```python
from build123d import *

# Parameters (mm, degrees)
F1_DEPTH = 520.7
F2_W     = 1016
F2_H     = 53.34
F3_DEPTH = 7.62
F4_R     = 7.62
F5_DEPTH = 10.16
F6_R     = 7.62
F7_DEPTH = 19.05
F8_R     = 7.62
F9_DEPTH = 19.05
F10_SIZE = 5.08


with BuildPart() as f1:
    # F0 (on Right) → F1 (new body, symmetric)
    with BuildSketch(Plane.YZ):
        Polygon((41.91, 39.37), (0, 39.37), (0, 0), (0, -39.37), (41.91, -39.37), (86.868, -26.67), (86.868, 0), (86.868, 26.67), align=None)
    extrude(amount=F1_DEPTH, both=True)

    # F2 (on face) → F3 (cut)
    with BuildSketch(Plane.XZ):
        Rectangle(F2_W, F2_H)
    extrude(amount=-F3_DEPTH, mode=Mode.SUBTRACT)

    # F4 (on face) → F5 (cut)
    with BuildSketch(Plane.XZ.offset(-7.62)):
        with Locations((-488.95, 13.97)):
            Circle(F4_R)
        with Locations((-463.8758824825, 13.97)):
            Circle(F4_R)
        with Locations((-438.8017649651, 13.97)):
            Circle(F4_R)
        with Locations((-413.7276474476, 13.97)):
            Circle(F4_R)
        with Locations((-388.6535299301, 13.97)):
            Circle(F4_R)
        with Locations((-363.5794124126, 13.97)):
            Circle(F4_R)
        with Locations((-338.5052948952, 13.97)):
            Circle(F4_R)
        with Locations((-313.4311773777, 13.97)):
            Circle(F4_R)
        with Locations((-288.3570598602, 13.97)):
            Circle(F4_R)
        with Locations((-263.2829423428, 13.97)):
            Circle(F4_R)
        with Locations((-238.2088248253, 13.97)):
            Circle(F4_R)
        with Locations((-213.1347073078, 13.97)):
            Circle(F4_R)
        with Locations((-188.0605897903, 13.97)):
            Circle(F4_R)
        with Locations((-162.9864722729, 13.97)):
            Circle(F4_R)
        with Locations((-137.9123547554, 13.97)):
            Circle(F4_R)
        with Locations((-112.8382372379, 13.97)):
            Circle(F4_R)
        with Locations((-87.7641197205, 13.97)):
            Circle(F4_R)
        with Locations((-62.690002203, 13.97)):
            Circle(F4_R)
        with Locations((-37.6158846855, 13.97)):
            Circle(F4_R)
        with Locations((-12.541767168, 13.97)):
            Circle(F4_R)
        with Locations((12.5323503494, 13.97)):
            Circle(F4_R)
        with Locations((37.6064678669, 13.97)):
            Circle(F4_R)
        with Locations((62.6805853844, 13.97)):
            Circle(F4_R)
        with Locations((87.7547029018, 13.97)):
            Circle(F4_R)
        with Locations((112.8288204193, 13.97)):
            Circle(F4_R)
        with Locations((137.9029379368, 13.97)):
            Circle(F4_R)
        with Locations((162.9770554543, 13.97)):
            Circle(F4_R)
        with Locations((188.0511729717, 13.97)):
            Circle(F4_R)
        with Locations((213.1252904892, 13.97)):
            Circle(F4_R)
        with Locations((238.1994080067, 13.97)):
            Circle(F4_R)
        with Locations((263.2735255241, 13.97)):
            Circle(F4_R)
        with Locations((288.3476430416, 13.97)):
            Circle(F4_R)
        with Locations((313.4217605591, 13.97)):
            Circle(F4_R)
        with Locations((338.4958780766, 13.97)):
            Circle(F4_R)
        with Locations((363.569995594, 13.97)):
            Circle(F4_R)
        with Locations((388.6441131115, 13.97)):
            Circle(F4_R)
        with Locations((413.718230629, 13.97)):
            Circle(F4_R)
        with Locations((438.7923481464, 13.97)):
            Circle(F4_R)
        with Locations((463.8664656639, 13.97)):
            Circle(F4_R)
        with Locations((488.9405831814, 13.97)):
            Circle(F4_R)
        with Locations((488.9405831814, -13.97)):
            Circle(F4_R)
        with Locations((-413.7276474476, -13.97)):
            Circle(F4_R)
        with Locations((-313.4311773777, -13.97)):
            Circle(F4_R)
        with Locations((12.5323503494, -13.97)):
            Circle(F4_R)
        with Locations((-37.6158846855, -13.97)):
            Circle(F4_R)
        with Locations((-87.7641197205, -13.97)):
            Circle(F4_R)
        with Locations((-388.6535299301, -13.97)):
            Circle(F4_R)
        with Locations((413.718230629, -13.97)):
            Circle(F4_R)
        with Locations((363.569995594, -13.97)):
            Circle(F4_R)
        with Locations((313.4217605591, -13.97)):
            Circle(F4_R)
        with Locations((-288.3570598602, -13.97)):
            Circle(F4_R)
        with Locations((-488.95, -13.97)):
            Circle(F4_R)
        with Locations((238.1994080067, -13.97)):
            Circle(F4_R)
        with Locations((162.9770554543, -13.97)):
            Circle(F4_R)
        with Locations((62.6805853844, -13.97)):
            Circle(F4_R)
        with Locations((-363.5794124126, -13.97)):
            Circle(F4_R)
        with Locations((112.8288204193, -13.97)):
            Circle(F4_R)
        with Locations((-263.2829423428, -13.97)):
            Circle(F4_R)
        with Locations((-188.0605897903, -13.97)):
            Circle(F4_R)
        with Locations((463.8664656639, -13.97)):
            Circle(F4_R)
        with Locations((-238.2088248253, -13.97)):
            Circle(F4_R)
        with Locations((-463.8758824825, -13.97)):
            Circle(F4_R)
        with Locations((37.6064678669, -13.97)):
            Circle(F4_R)
        with Locations((-162.9864722729, -13.97)):
            Circle(F4_R)
        with Locations((-62.690002203, -13.97)):
            Circle(F4_R)
        with Locations((-112.8382372379, -13.97)):
            Circle(F4_R)
        with Locations((-12.541767168, -13.97)):
            Circle(F4_R)
        with Locations((438.7923481464, -13.97)):
            Circle(F4_R)
        with Locations((388.6441131115, -13.97)):
            Circle(F4_R)
        with Locations((338.4958780766, -13.97)):
            Circle(F4_R)
        with Locations((288.3476430416, -13.97)):
            Circle(F4_R)
        with Locations((213.1252904892, -13.97)):
            Circle(F4_R)
        with Locations((263.2735255241, -13.97)):
            Circle(F4_R)
        with Locations((-213.1347073078, -13.97)):
            Circle(F4_R)
        with Locations((-438.8017649651, -13.97)):
            Circle(F4_R)
        with Locations((-137.9123547554, -13.97)):
            Circle(F4_R)
        with Locations((-338.5052948952, -13.97)):
            Circle(F4_R)
        with Locations((137.9029379368, -13.97)):
            Circle(F4_R)
        with Locations((87.7547029018, -13.97)):
            Circle(F4_R)
        with Locations((188.0511729717, -13.97)):
            Circle(F4_R)
    extrude(amount=-F5_DEPTH, mode=Mode.SUBTRACT)

    # F6 (on face) → F7 (cut)
    with BuildSketch(Plane.YZ.offset(520.7)):
        with Locations((41.91, 0)):
            Circle(F6_R)
    extrude(amount=-F7_DEPTH, mode=Mode.SUBTRACT)

    # F8 (on face) → F9 (cut)
    with BuildSketch(Plane(origin=(-520.7, 0, 0), x_dir=(0, -1, 0), z_dir=(-1, 0, 0))):
        with Locations((-41.91, 0)):
            Circle(F8_R)
    extrude(amount=-F9_DEPTH, mode=Mode.SUBTRACT)

    # F10
    f10_edges = [f1.edges().sort_by_distance(p)[0] for p in [
        (-520.7, 20.955, 39.37),
        (-520.7, 64.389, 33.02),
        (-520.7, 0, 0),
        (-520.7, 86.868, 0),
        (-520.7, 20.955, -39.37),
        (-520.7, 64.389, -33.02),
        (-520.7, 49.53, 0),
        (520.7, 20.955, 39.37),
        (520.7, 64.389, 33.02),
        (520.7, 0, 0),
        (520.7, 86.868, 0),
        (520.7, 20.955, -39.37),
        (520.7, 64.389, -33.02),
        (520.7, 34.29, 0),
        (0, 0, 39.37),
        (0, 0, -39.37),
    ]]
    chamfer(f10_edges, length=F10_SIZE)


solid = f1.part
```
The listing builds one solid part. Answer for the finished solid, in the listing's coordinates (mm). A direction names the side the tool comes from. Coordinates: 2 decimals unless noted, no trailing zeros.
Q1. Which of the six approach directions +Z, -Z, +X, -X, +Y, -Y give full straight-line access (tool end or side, diameter ignored) to faces 4 (the flat face through (-7, 7.62, 0)), 5 (the flat face through (518.124, 63.393, -30.699))?
Returned:
face 4: -Y
face 5: -Z, +X, +Y
Q2. The mould has two halves that part along Z. Classify faces 1 (the flat face through (-520.7, 26, 0)), 2 (the conical face through (-515.87, 49.77, 0.35)), 3 (the flat face through (7.219, 64.704, 32.931)): released by +Z, released by -Z, zero draft, split by the parting line, or undercut.
Returned:
face 1: zero draft
face 2: undercut
face 3: released by +Z
Q3. Given P1, Ø3, axis at x = 267.5, y = 52, coming from the -Z side; P2, Ø17.5, axis at x = -188.06, z = -13.97, coming from the -Y side; P3, Ø7.5, axis at x = -389.5, z = -14.5, coming from the -Y side, each flat-ended and moving along its own axis, determine where each tip first touches the part or whether it passes through.
Returned:
P1: stops at z = -36.94
P2: stops at y = 7.62
P3: stops at y = 17.78
Q4. Find the intervals of material crossed by line 1 along Y through (x, z) = (-268, -23.5); line 2 along Y through (x, z) = (264, -21.5); line 3 along Z through (x, y) = (-283.5, 62), in increasing order.
Returned:
line 1: y = 7.62 to 86.87
line 2: y = 17.78 to 86.87
line 3: z = -33.69 to 33.69
